Source: CAD feature listing. Evaluate the final solid. Frame: model axes, mm. Give positions to 0.01 mm unless a question says otherwise; leave off trailing zeros. Loops run counter-clockwise (first coordinate to the right, second up) from the corner with the lowest first, then second, coordinate; pieces in that order, holes last. Notation, with made-up numbers: (22, 59.25) -> (35, 59.25) arc R17 cw to (35, 89.25) -> close; hole circle Ø4 at (63, 85). An arc over 180 degrees is marked (long way). Return JSON: item names as keys, results as strings. Group by question number.
(1) Cut plane C-C on z = -29.72. Return loops of the section in (x, y), then the cut area to 3 significant figures.
(2) Cut plane D-D on z = -16. Return loops of the section in (x, y).
(3) Ray query, line 1 (X direction, y = 0.5, z = 29.72); line 2 (X direction, y = 1.4, z = -0.5); line 3 (Z direction, x = -26.42, y = 0.9). Return the intervals inside material, ascending. Write a range as from..to.
(4) Cut plane B-B on y = 0.35. Return loops of the section in (x, z), then the cut area to 3 significant figures.
(5) Pin query (flat end, axial travel): pin 1 (12 mm diameter, centred on x = 38, z = -27.5, fed in from -Y). Return the tip coordinate at first contact, or that it passes through.
(6) Cut plane A-A on x = 26.42. Return loops of the section in (y, z).
(7) Draft query along X for faces 1 (the face through (26.496, 0.805, -31.446)), 2 (the face through (1, 1.588, -1)), 3 (the face through (2.19, 0.78, -49.73)). Return one class per face: released by +X, released by -X, zero draft, split by the parting line, or undercut.
```python
from build123d import *

# Parameters (mm, degrees)
SKETCH1_R      = 49.78
EXTRUDE1_DEPTH = 1.5875
SKETCH2_R      = 1.7272
EXTRUDE2_DEPTH = 10


with BuildPart() as part:
    # Sketch1 → Extrude1 (new body)
    with BuildSketch(Plane(origin=(0, 0, 0), x_dir=(1, 0, 0), z_dir=(0, 1, 0))):
        with Locations(Location((0, 0, 0), (0, 0, 270))):
            Circle(SKETCH1_R)
    extrude(amount=EXTRUDE1_DEPTH)

    # Sketch2 → Extrude2 (cut)
    with BuildSketch(Plane(origin=(0, 1.5875, 0), x_dir=(-1, 0, 0), z_dir=(0, 1, 0))):
        with Locations(Location((-26.42, -29.72, 0), (0, 0, 90))):
            Circle(SKETCH2_R)
        with Locations(Location((-26.42, 29.72, 0), (0, 0, 90))):
            Circle(SKETCH2_R)
    extrude2 = extrude(amount=-EXTRUDE2_DEPTH, mode=Mode.SUBTRACT)

    # Mirror1: Extrude2 across plane
    add(extrude2.mirror(Plane(origin=(0, 0, 0), x_dir=(0, 0, 1), z_dir=(1, 0, 0))), mode=Mode.SUBTRACT)


solid = part.part
```
Answers:
{
 "1": {"outline": "(-39.93, 0) -> (-28.15, 0) -> (-28.15, 1.59) -> (-39.93, 1.59) -> close; (-24.69, 0) -> (24.69, 0) -> (24.69, 1.59) -> (-24.69, 1.59) -> close; (28.15, 0) -> (39.93, 0) -> (39.93, 1.59) -> (28.15, 1.59) -> close", "area": "116 mm²"},
 "2": {"outline": "(-47.14, 0) -> (47.14, 0) -> (47.14, 1.59) -> (-47.14, 1.59) -> close"},
 "3": {"line 1": "-39.93..-28.15, -24.69..24.69, 28.15..39.93", "line 2": "-49.78..49.78", "line 3": "-42.19..-31.45, -27.99..27.99, 31.45..42.19"},
 "4": {"outline": "circle Ø99.56 at (0, 0); hole circle Ø3.45 at (-26.42, -29.72); hole circle Ø3.45 at (-26.42, 29.72); hole circle Ø3.45 at (26.42, -29.72); hole circle Ø3.45 at (26.42, 29.72)", "area": "7,750 mm²"},
 "5": {"pin 1": "y = 0"},
 "6": {"outline": "(0, -42.19) -> (1.59, -42.19) -> (1.59, -31.45) -> (0, -31.45) -> close; (0, -27.99) -> (1.59, -27.99) -> (1.59, 27.99) -> (0, 27.99) -> close; (0, 31.45) -> (1.59, 31.45) -> (1.59, 42.19) -> (0, 42.19) -> close"},
 "7": {"face 1": "undercut", "face 2": "zero draft", "face 3": "split by the parting line"}
}
